The model under review builds one solid part; all positions refer to its coordinate system, in mm. A direction names the side the tool comes from. Round coordinates to 2 decimals unless told otherwise and drop trailing zeros. Order: outer loops, then holes, each group sorted by start corner. A loop starts at its lowest first (then second) coordinate and runs counter-clockwise, first axis right, second up.
1) Clearance check with flat-ended pins moving along their axes: P1, Ø2, axis at x = 23, y = -3.5, coming from the -Z side; P2, Ø4.5, axis at x = 11, y = -1.5, coming from the -Z side; P3, Ø1.2, axis at x = -21.5, y = -1, coming from the -Z side. State where each tip first meets the part, or that it passes through.
2) Consider section C-C (y = -6.5). Give the boundary of the cut face in (x, z), then the cut area to 3 significant figures.
3) Consider section D-D (x = 8.5). Give the boundary of the cut face in (y, z) (3 decimals).
4) To check wall thickness, follow L1, parallel to X at y = -2, z = 18.6 (3 decimals); L2, parallel to X at y = -2, z = 19.5 (3 decimals); L3, parallel to X at y = 8.25, z = 15.5. State the ranges of each line that lie inside material, in increasing order.
5) Consider section A-A (x = -5). Give the boundary of the cut face in (y, z), then the cut area to 3 significant figures.
6) Machinability: for faces 4 (the face through (0, 10, 9)), 5 (the face through (-6.8, -2.5, 18)), which of the approach directions +Z, -Z, +X, -X, +Y, -Y give a long, thin tool a straight path to every point of the face, cutting with its end or side? Answer none if there is none.
7) Consider section B-B (z = 3.5). Give the boundary of the cut face in (x, y), then the cut area to 3 significant figures.
8) Mouldability with a two-part tool opening along X and no side actions: class faces 1 (the face through (29.5, -9.5, 9.6)), 2 (the face through (0, 2, 20)), 3 (the face through (-23.905, -2.05, 17.493)) as pulls with the +X half, pulls with the -X half, needs draft (parallel to the pull), parting line crosses it, or undercut.
from build123d import *

# Parameters (mm, degrees)
SKETCH001_W            = 60
SKETCH001_H            = 20
PAD_DEPTH              = 20
SKETCH002_W            = 50
SKETCH002_H            = 17
POCKET_DEPTH           = 17
POCKET001_DEPTH        = 1
LINEARPATTERN_COUNT    = 5
LINEARPATTERN_PITCH    = 10
SKETCH004_R            = 3.075
POCKET002_DEPTH        = 2.001
LINEARPATTERN001_COUNT = 5
LINEARPATTERN001_PITCH = 10
CHAMFER_SIZE           = 1
CHAMFER001_SIZE        = 1


with BuildPart() as part:
    # Sketch001 → Pad (new body)
    with BuildSketch(Plane.XY):
        Rectangle(SKETCH001_W, SKETCH001_H)
    extrude(amount=PAD_DEPTH)

    # Sketch002 → Pocket (cut)
    with BuildSketch(Plane.XY):
        Rectangle(SKETCH002_W, SKETCH002_H)
    extrude(amount=POCKET_DEPTH, mode=Mode.SUBTRACT)

    # Sketch003 (on Face11 of Pocket) → Pocket001 (cut)
    with BuildSketch(Plane(origin=(0, 0, 17), x_dir=(1, 0, 0), z_dir=(0, 0, -1))):
        with BuildLine():
            ThreePointArc((-22.407381, 5.075), (-23.905267, 2), (-22.407381, -1.075))
            Line((-22.407381, -1.075), (-17.592619, -1.075))
            ThreePointArc((-17.592619, -1.075), (-16.094733, 2), (-17.592619, 5.075))
            Line((-22.407381, 5.075), (-17.592619, 5.075))
        make_face()
    pocket001 = extrude(amount=-POCKET001_DEPTH, mode=Mode.SUBTRACT)

    # LinearPattern: Pocket001 ×5
    with Locations(*[(i * LINEARPATTERN_PITCH, 0, 0) for i in range(1, LINEARPATTERN_COUNT)]):
        add(pocket001, mode=Mode.SUBTRACT)

    # Sketch004 (on Face16 of Pocket001) → Pocket002 (cut, through all)
    with BuildSketch(Plane(origin=(0, 0, 18), x_dir=(1, 0, 0), z_dir=(0, 0, -1))):
        with Locations((-20, 2)):
            Circle(SKETCH004_R)
    pocket002 = extrude(amount=-POCKET002_DEPTH, mode=Mode.SUBTRACT)

    # LinearPattern001: Pocket002 ×5
    with Locations(*[(i * LINEARPATTERN001_PITCH, 0, 0) for i in range(1, LINEARPATTERN001_COUNT)]):
        add(pocket002, mode=Mode.SUBTRACT)

    # Chamfer
    chamfer_edges = [part.edges().sort_by_distance(p)[0] for p in [
        (0, 10, 20),
        (-30, 0, 20),
        (0, -10, 20),
        (30, 0, 20),
    ]]
    chamfer(chamfer_edges, length=CHAMFER_SIZE)

    # Chamfer001
    chamfer001_edges = [part.edges().sort_by_distance(p)[0] for p in [
        (-30, -10, 9.5),
        (-30, 10, 9.5),
        (30, -10, 9.5),
        (30, 10, 9.5),
    ]]
    chamfer(chamfer001_edges, length=CHAMFER001_SIZE)


solid = part.part
Answer below:
1. P1: stops at z = 17
1. P2: stops at z = 18
1. P3: passes through
2. outline: (-30, 0) - (-25, 0) - (-25, 17) - (25, 17) - (25, 0) - (30, 0) - (30, 19) - (29, 20) - (-29, 20) - (-30, 19) - close
2. area: 349 mm2
3. outline: (-10, 0) - (-8.5, 0) - (-8.5, 17) - (-5.075, 17) - (-5.075, 18) - (-4.684, 18) - (-4.684, 20) - (-9, 20) - (-10, 19) - close; (0.684, 18) - (1.075, 18) - (1.075, 17) - (8.5, 17) - (8.5, 0) - (10, 0) - (10, 19) - (9, 20) - (0.684, 20) - close
4. L1: x = -30 to -23.075, -16.925 to -13.075, -6.925 to -3.075, 3.075 to 6.925, 13.075 to 16.925, 23.075 to 30
4. L2: x = -29.5 to -23.075, -16.925 to -13.075, -6.925 to -3.075, 3.075 to 6.925, 13.075 to 16.925, 23.075 to 29.5
4. L3: x = -30 to -25, 25 to 30
5. outline: (-10, 0) - (-8.5, 0) - (-8.5, 17) - (8.5, 17) - (8.5, 0) - (10, 0) - (10, 19) - (9, 20) - (-9, 20) - (-10, 19) - close
5. area: 110 mm2
6. face 4: +Z, -Z, +X, -X, +Y
6. face 5: -Z
7. outline: (-30, -9) - (-29, -10) - (29, -10) - (30, -9) - (30, 9) - (29, 10) - (-29, 10) - (-30, 9) - close; hole (-25, -8.5) - (25, -8.5) - (25, 8.5) - (-25, 8.5) - close
7. area: 348 mm2
8. face 1: pulls with the +X half
8. face 2: needs draft
8. face 3: undercut
